Part print with two shaded views. Sizes in mm from the minimum x, y, z corner. A direction names the side the tool comes from. Give positions to 0.01 mm unless a question says otherwise; leave off trailing zeros. Loops run counter-clockwise (first coordinate to the right, second up) from the corner with the lowest first, then second, coordinate; pieces in that order, holes last. Notation, with made-up numbers: M 38.25,22 L 55.25,22 A30 ccw 55.25,59 Z; hole C 74.25,20.5 d1. An arc over 180 degrees is marked long. Answer in a Markdown table with one row per item.
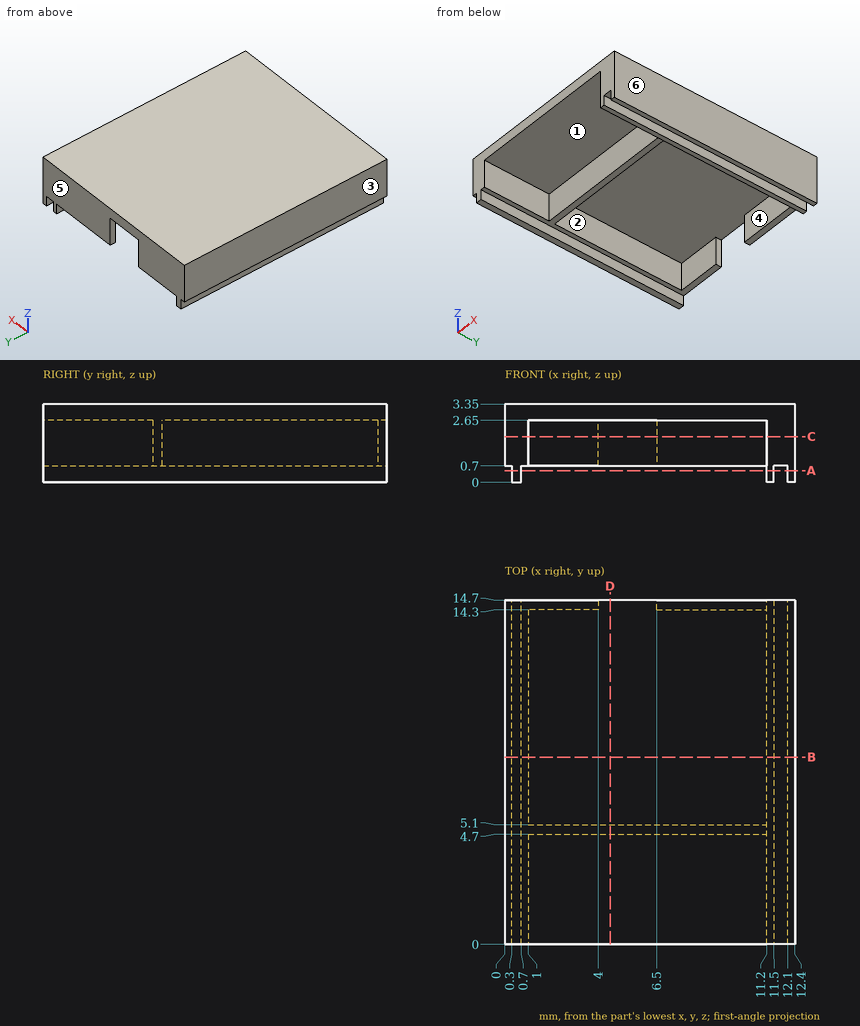
Q1. Saw through at B-B (y = 8). Give the cut face in (x, z).
Reported:
| item | result |
|---|---|
| outline | M 0,0.7 L 0.3,0.7 L 0.3,0 L 0.7,0 L 0.7,0.7 L 1,0.7 L 1,2.65 L 11.2,2.65 L 11.2,0 L 11.5,0 L 11.5,0.7 L 12.1,0.7 L 12.1,0 L 12.4,0 L 12.4,3.35 L 0,3.35 Z |
Q2. Saw through at D-D (x = 4.5). Give the cut face in (y, z).
Reported:
| item | result |
|---|---|
| outline | M 0,2.65 L 4.7,2.65 L 4.7,0.7 L 5.1,0.7 L 5.1,2.65 L 14.7,2.65 L 14.7,3.35 L 0,3.35 Z |
Q3. 3-axis set-ups, long thin cutter, end or side, ignore diameter. For the marked faces 1, 2 and 3: which of +Z, -Z, +X, -X, +Y, -Y reach the whole face in a straight line?
Reported:
| item | result |
|---|---|
| face 1 | -Z, -Y |
| face 2 | -Z |
| face 3 | +Z, -Z, -X, +Y, -Y |
Q4. Mould opens along Y. For the marked faces 4, 5 and 6 say: released by +Y, released by -Y, zero draft, split by the parting line, or undercut.
Reported:
| item | result |
|---|---|
| face 4 | undercut |
| face 5 | released by +Y |
| face 6 | zero draft |
Q5. Saw through at A-A (z = 0.5). Give the cut face in (x, y).
Reported:
| item | result |
|---|---|
| outline | M 0.3,0 L 0.7,0 L 0.7,14.7 L 0.3,14.7 Z; M 11.2,0 L 11.5,0 L 11.5,14.7 L 11.2,14.7 Z; M 12.1,0 L 12.4,0 L 12.4,14.7 L 12.1,14.7 Z |
Q6. Saw through at C-C (z = 1.95). Give the cut face in (x, y).
Reported:
| item | result |
|---|---|
| outline | M 0,0 L 1,0 L 1,4.7 L 11.2,4.7 L 11.2,0 L 12.4,0 L 12.4,14.7 L 6.5,14.7 L 6.5,14.3 L 11.2,14.3 L 11.2,5.1 L 1,5.1 L 1,14.3 L 4,14.3 L 4,14.7 L 0,14.7 Z |
Q7. Drop flat-ended pins along their axis: pin 1 (2 mm diameter, centred on x = 9, z = 1.5, fed in from -Y); pin 2 (2 mm diameter, centred on x = 8, y = 8, fed in from -Z). Give the stop position or say it passes through.
Reported:
| item | result |
|---|---|
| pin 1 | y = 4.7 |
| pin 2 | z = 2.65 |
Q8. Probe probe 1 along X at (y, z) = (9.25, 0.6); probe 2 along X at (y, z) = (10.5, 2.1); probe 3 along Y at (x, z) = (2.25, 2.2). List the from-to ranges inside material, lowest first.
Reported:
| item | result |
|---|---|
| probe 1 | 0.3 to 0.7, 11.2 to 11.5, 12.1 to 12.4 |
| probe 2 | 0 to 1, 11.2 to 12.4 |
| probe 3 | 4.7 to 5.1, 14.3 to 14.7 |
